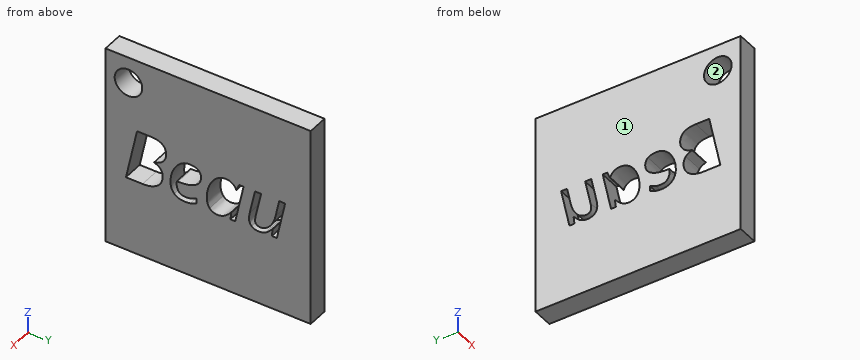
from build123d import *

# Parameters (mm, degrees)
F0_W     = 50
F0_H     = 48.9445883323
F0_R     = 3.3555723101
F1_DEPTH = 5


with BuildPart() as f1:
    # F0 (on Right) → F1 (new body)
    with BuildSketch(Plane.YZ):
        with Locations((1.9210092723, -2.0170593634)):
            Rectangle(F0_W, F0_H)
        with BuildLine():
            add(Edge.make_bspline(
                [(-2.4102224398, -8.1740687344), (-3.0415094863, -8.3283833458), (-3.8018596622, -8.3283833458)],
                knots=[0, 0, 0, 1, 1, 1], degree=2))
            add(Edge.make_bspline(
                [(-3.8018596622, -8.3283833458), (-5.415148781, -8.3283833458), (-6.3368278688, -7.3716327553)],
                knots=[0, 0, 0, 1, 1, 1], degree=2))
            add(Edge.make_bspline(
                [(-6.3368278688, -7.3716327553), (-7.2585069566, -6.4148821649), (-7.2585069566, -4.7230328804)],
                knots=[0, 0, 0, 1, 1, 1], degree=2))
            add(Edge.make_bspline(
                [(-7.2585069566, -4.7230328804), (-7.2585069566, -3.0760751192), (-6.6047741485, -1.5623890678)],
                knots=[0, 0, 0, 1, 1, 1], degree=2))
            add(Edge.make_bspline(
                [(-6.6047741485, -1.5623890678), (-5.9510413404, -0.0487030164), (-4.872241921, 0.7930130455)],
                knots=[0, 0, 0, 1, 1, 1], degree=2))
            add(Edge.make_bspline(
                [(-4.872241921, 0.7930130455), (-3.7934425016, 1.6347291075), (-2.4971997662, 1.6347291075)],
                knots=[0, 0, 0, 1, 1, 1], degree=2))
            add(Edge.make_bspline(
                [(-2.4971997662, 1.6347291075), (-1.1560655075, 1.6347291075), (-0.4798869378, 1.0511393045)],
                knots=[0, 0, 0, 1, 1, 1], degree=2))
            add(Edge.make_bspline(
                [(-0.4798869378, 1.0511393045), (0.196291632, 0.4675495016), (0.196291632, -0.5761784152)],
                knots=[0, 0, 0, 1, 1, 1], degree=2))
            add(Edge.make_bspline(
                [(0.196291632, -0.5761784152), (0.196291632, -2.1529931713), (-1.2598771552, -3.0522264975)],
                knots=[0, 0, 0, 1, 1, 1], degree=2))
            add(Edge.make_bspline(
                [(-1.2598771552, -3.0522264975), (-2.7160459423, -3.9514598236), (-5.4263716618, -3.9514598236)],
                knots=[0, 0, 0, 1, 1, 1], degree=2))
            Line((-5.4263716618, -3.9514598236), (-5.7153608431, -3.9514598236))
            Line((-5.7153608431, -3.9514598236), (-5.7490294855, -4.6528898753))
            add(Edge.make_bspline(
                [(-5.7490294855, -4.6528898753), (-5.7490294855, -5.8004294397), (-5.2103312059, -6.4457450872)],
                knots=[0, 0, 0, 1, 1, 1], degree=2))
            add(Edge.make_bspline(
                [(-5.2103312059, -6.4457450872), (-4.6716329263, -7.0910607347), (-3.540927683, -7.0910607347)],
                knots=[0, 0, 0, 1, 1, 1], degree=2))
            add(Edge.make_bspline(
                [(-3.540927683, -7.0910607347), (-2.9882008024, -7.0910607347), (-2.4046109994, -6.932537543)],
                knots=[0, 0, 0, 1, 1, 1], degree=2))
            add(Edge.make_bspline(
                [(-2.4046109994, -6.932537543), (-1.8210211965, -6.7740143514), (-0.9540536527, -6.3531563204)],
                knots=[0, 0, 0, 1, 1, 1], degree=2))
            Line((-0.9540536527, -6.3531563204), (-0.9540536527, -7.6353704547))
            add(Edge.make_bspline(
                [(-0.9540536527, -7.6353704547), (-1.7789353934, -8.019754123), (-2.4102224398, -8.1740687344)],
                knots=[0, 0, 0, 1, 1, 1], degree=2))
        make_face(mode=Mode.SUBTRACT)
        with BuildLine():
            add(Edge.make_bspline(
                [(3.9377195273, 0.7481215222), (5.033353268, 1.6347291075), (6.3408188842, 1.6347291075)],
                knots=[0, 0, 0, 1, 1, 1], degree=2))
            add(Edge.make_bspline(
                [(6.3408188842, 1.6347291075), (7.1460605834, 1.6347291075), (7.7773476299, 1.1998424755)],
                knots=[0, 0, 0, 1, 1, 1], degree=2))
            add(Edge.make_bspline(
                [(7.7773476299, 1.1998424755), (8.4086346764, 0.7649558435), (8.7593497022, -0.0487030164)],
                knots=[0, 0, 0, 1, 1, 1], degree=2))
            Line((8.7593497022, -0.0487030164), (8.8575499094, -0.0487030164))
            Line((8.8575499094, -0.0487030164), (9.4439454326, 1.4579687345))
            Line((9.4439454326, 1.4579687345), (10.5578163545, 1.4579687345))
            Line((10.5578163545, 1.4579687345), (8.5152520442, -8.1516229727))
            Line((8.5152520442, -8.1516229727), (7.3480724383, -8.1516229727))
            Line((7.3480724383, -8.1516229727), (7.5781414952, -6.3194876779))
            Line((7.5781414952, -6.3194876779), (7.5079984901, -6.3194876779))
            add(Edge.make_bspline(
                [(7.5079984901, -6.3194876779), (5.9367951745, -8.3283833458), (4.2000543666, -8.3283833458)],
                knots=[0, 0, 0, 1, 1, 1], degree=2))
            add(Edge.make_bspline(
                [(4.2000543666, -8.3283833458), (2.982371797, -8.3283833458), (2.289358906, -7.4600129418)],
                knots=[0, 0, 0, 1, 1, 1], degree=2))
            add(Edge.make_bspline(
                [(2.289358906, -7.4600129418), (1.596346015, -6.5916425379), (1.596346015, -5.0821650669)],
                knots=[0, 0, 0, 1, 1, 1], degree=2))
            add(Edge.make_bspline(
                [(1.596346015, -5.0821650669), (1.596346015, -3.2584469326), (2.2192159009, -1.6984664978)],
                knots=[0, 0, 0, 1, 1, 1], degree=2))
            add(Edge.make_bspline(
                [(2.2192159009, -1.6984664978), (2.8420857867, -0.138486063), (3.9377195273, 0.7481215222)],
                knots=[0, 0, 0, 1, 1, 1], degree=2))
        make_face(mode=Mode.SUBTRACT)
        with BuildLine():
            Line((13.3467022398, 1.4579687345), (14.8365396694, 1.4579687345))
            Line((14.8365396694, 1.4579687345), (13.5234626128, -4.636055554))
            add(Edge.make_bspline(
                [(13.5234626128, -4.636055554), (13.363536561, -5.4160457714), (13.363536561, -5.8537381236)],
                knots=[0, 0, 0, 1, 1, 1], degree=2))
            add(Edge.make_bspline(
                [(13.363536561, -5.8537381236), (13.363536561, -7.1078950559), (14.654167856, -7.1078950559)],
                knots=[0, 0, 0, 1, 1, 1], degree=2))
            add(Edge.make_bspline(
                [(14.654167856, -7.1078950559), (15.4257409128, -7.1078950559), (16.1706596276, -6.5818225172)],
                knots=[0, 0, 0, 1, 1, 1], degree=2))
            add(Edge.make_bspline(
                [(16.1706596276, -6.5818225172), (16.9155783424, -6.0557499785), (17.4851395443, -5.0737479062)],
                knots=[0, 0, 0, 1, 1, 1], degree=2))
            add(Edge.make_bspline(
                [(17.4851395443, -5.0737479062), (18.0547007462, -4.091745834), (18.3549128083, -2.705720052)],
                knots=[0, 0, 0, 1, 1, 1], degree=2))
            Line((18.3549128083, -2.705720052), (19.2302975128, 1.4579687345))
            Line((19.2302975128, 1.4579687345), (20.6864662999, 1.4579687345))
            Line((20.6864662999, 1.4579687345), (18.6607363108, -8.1516229727))
            Line((18.6607363108, -8.1516229727), (17.4430537412, -8.1516229727))
            Line((17.4430537412, -8.1516229727), (17.6338427153, -6.3727963618))
            Line((17.6338427153, -6.3727963618), (17.5300310676, -6.3727963618))
            add(Edge.make_bspline(
                [(17.5300310676, -6.3727963618), (16.6714806845, -7.4670272424), (15.8900876069, -7.8977052941)],
                knots=[0, 0, 0, 1, 1, 1], degree=2))
            add(Edge.make_bspline(
                [(15.8900876069, -7.8977052941), (15.1086945294, -8.3283833458), (14.2753956281, -8.3283833458)],
                knots=[0, 0, 0, 1, 1, 1], degree=2))
            add(Edge.make_bspline(
                [(14.2753956281, -8.3283833458), (13.1531075455, -8.3283833458), (12.5134033384, -7.7181392008)],
                knots=[0, 0, 0, 1, 1, 1], degree=2))
            add(Edge.make_bspline(
                [(12.5134033384, -7.7181392008), (11.8736991314, -7.1078950559), (11.8736991314, -5.9771898127)],
                knots=[0, 0, 0, 1, 1, 1], degree=2))
            add(Edge.make_bspline(
                [(11.8736991314, -5.9771898127), (11.8736991314, -5.4328800927), (12.0672938256, -4.4677123416)],
                knots=[0, 0, 0, 1, 1, 1], degree=2))
            Line((12.0672938256, -4.4677123416), (13.3467022398, 1.4579687345))
        make_face(mode=Mode.SUBTRACT)
        with BuildLine():
            Line((-15.3950955554, 4.6677126507), (-12.1067914734, 4.6677126507))
            add(Edge.make_bspline(
                [(-12.1067914734, 4.6677126507), (-8.3190691947, 4.6677126507), (-8.3190691947, 1.7217064339)],
                knots=[0, 0, 0, 1, 1, 1], degree=2))
            add(Edge.make_bspline(
                [(-8.3190691947, 1.7217064339), (-8.3190691947, 0.4843838228), (-9.0808222307, -0.3657493998)],
                knots=[0, 0, 0, 1, 1, 1], degree=2))
            add(Edge.make_bspline(
                [(-9.0808222307, -0.3657493998), (-9.8425752668, -1.2158826223), (-11.2286010488, -1.4712031611)],
                knots=[0, 0, 0, 1, 1, 1], degree=2))
            Line((-11.2286010488, -1.4712031611), (-11.2286010488, -1.5581804875))
            add(Edge.make_bspline(
                [(-11.2286010488, -1.5581804875), (-10.2213474947, -1.8387525082), (-9.6812463549, -2.5275568188)],
                knots=[0, 0, 0, 1, 1, 1], degree=2))
            add(Edge.make_bspline(
                [(-9.6812463549, -2.5275568188), (-9.1411452152, -3.2163611295), (-9.1411452152, -4.1787231604)],
                knots=[0, 0, 0, 1, 1, 1], degree=2))
            add(Edge.make_bspline(
                [(-9.1411452152, -4.1787231604), (-9.1411452152, -6.0389156573), (-10.4738623133, -7.095269315)],
                knots=[0, 0, 0, 1, 1, 1], degree=2))
            add(Edge.make_bspline(
                [(-10.4738623133, -7.095269315), (-11.8065794113, -8.1516229727), (-14.0427384159, -8.1516229727)],
                knots=[0, 0, 0, 1, 1, 1], degree=2))
            Line((-14.0427384159, -8.1516229727), (-18.1026155547, -8.1516229727))
            Line((-18.1026155547, -8.1516229727), (-15.3950955554, 4.6677126507))
        make_face(mode=Mode.SUBTRACT)
        with Locations((-17.4894966185, 16.0714294761)):
            Circle(F0_R, mode=Mode.SUBTRACT)
    extrude(amount=F1_DEPTH)


solid = f1.part
Source: CAD feature listing. Evaluate the final solid. Frame: model axes, mm. Face numbers are marked on the shaded views. Give positions to 0.01 mm unless a question says otherwise; leave off trailing zeros. Write each loop counter-clockwise with the first axis right and the second up, starting at its lowest first coordinate (ties: lowest second). Pieces come first, ordered by that corner, then holes. Notation, with made-up numbers: (16, 51.5) - (25, 51.5) arc R29 ccw to (25, 74.5) - close; hole circle Ø7 at (-36, -30.5). An arc over 180 degrees is marked (long way). Write item = value, one per line. Start each with the question number.
Q1. Pin query (flat end, axial travel): pin 1 Ø2 at (y, z) = (12, -0.5) entering from -X. Return the tip coordinate at first contact, or that it passes through.
Q2. Material intervals for probe 1 along Z at (x, y) = (3.6, -11); probe 2 along Z at (x, y) = (0.95, -14); probe 3 along Y at (x, z) = (3.5, 16), sorted ascending.
Q3. Draft query along Y for the marked faces 1 and 2. Return one class per face: +Y half, -Y half, draft (parallel to the pull), parting line (faces both ways), or undercut.
Q4. Cut plane A-A, the plane y = 20. Return loops of the section in (x, z), then the cut area to 3 significant figures.
Q5. Cut plane B-B, the plane x = 3.7. Give the number of separate pieces and of enclosed holes in the cut face, then the cut area to 3 significant figures.
Computed values:
q1.pin_1 = 0
q2.probe_1 = -26.49 to -7.45, -1.63 to -1.42, 4.59 to 22.46
q2.probe_2 = -26.49 to -8.15, 4.67 to 22.46
q2.probe_3 = -23.08 to -20.84, -14.13 to 26.92
q3.face_1 = draft
q3.face_2 = undercut
q4.outline = (0, -26.49) - (5, -26.49) - (5, -1.8) - (0, -1.8) - close; (0, 1.46) - (5, 1.46) - (5, 22.46) - (0, 22.46) - close
q4.area = 228 mm²
q5.separate_pieces = 1
q5.enclosed_holes = 5
q5.area = 2,180 mm²
